Can you work these out from the model? Positions are in its coordinate system, mm. Face numbers are marked on the shaded views. Give positions to 0.01 mm unless a question says otherwise; leave off trailing zeros. Loops run counter-clockwise (first coordinate to the right, second up) from the corner with the lowest first, then second, coordinate; pieces in that order, holes last. Notation, with made-up numbers: M -1,52 L 45,52 A24 cw 45,91 Z; hole C 73,58 d3. An arc over 180 degrees is marked long. One line per item, written item: value. Start each with the question number.
Autodesk Inventor part; units mm, degrees
ref_plane "YZ Plane" through (0, 0, 0) normal (1, 0, 0) x (0, 1, 0)
ref_plane "XZ Plane" through (0, 0, 0) normal (0, 1, 0) x (-1, 0, 0)
ref_plane "XY Plane" through (0, 0, 0) normal (0, 0, 1) x (1, 0, 0)
sketch "Sketch1" plane through (0, 0, 0) normal (0, 1, 0) x (-1, 0, 0)
  circle A0 centre (0, 0) radius 1.05
  line L0 (5, 20) -> (-5, 20)
  line L1 (-5, 20) -> (-5, -5)
  line L2 (-5, -5) -> (5, -5)
  line L3 (5, -5) -> (5, 20)
  circle A1 centre (0, 15) radius 1.05
  dimension "d0" = 2.1
  dimension "d1" = 5
  dimension "d2" = 10
  dimension "d4" = 5
  dimension "d16" = 2.1
  dimension "d17" = 15
  dimension "d18" = 5
extrude "Extrusion1" add sketch "Sketch1" along normal blind 10
sketch "Sketch2" plane through (5, 0, 20) normal (1, 0, 0) x (0, 0, -1)
  line L0 (0, 10) -> (25, 10)
  line L1 (15, 10) -> (17.5478, 3)
  line L2 (17.5478, 3) -> (25, 3)
  line L3 (18.95, 10) -> (18.95, 0)
  line L4 (25, 3) -> (25, 10)
  line L5 (25, 10) -> (15, 10)
  line L6 (25, 0) -> (25, 10)
  line L7 (0, 0) -> (25, 0)
  point P0 (20, 0)
  dimension "d8" = 3
  dimension "d9" = 110
  dimension "d10" = 10
extrude "Extrusion2" cut sketch "Sketch2" against normal blind 10 contours L0 L3 L2 L1 | L0 L4 L2 L3
sketch "Sketch3" plane through (0, 10, 0) normal (0, 1, 0) x (1, 0, 0)
  circle A0 centre (0, 0) radius 2
  dimension "d13" = 4
extrude "Extrusion3" cut sketch "Sketch3" against normal up to surface (7 mm away)
sketch "Sketch4" plane through (0, 10, 0) normal (0, 1, 0) x (1, 0, 0)
  circle A0 centre (0, -15) radius 1.05
  circle A1 centre (0, -15) radius 2.25
  point P0 (0, 0)
  dimension "d19" = 4.5
extrude "Extrusion4" cut sketch "Sketch4" against normal up to surface (7 mm away)
chamfer "Chamfer1" distance 1 angle 45 1 edges at (1.05, 3, 0)
sketch "Sketch5" plane through (5, 0, -5) normal (0, 0, -1) x (-1, 0, 0)
  line L0 (5, 0) -> (5, 5.666) construction
  circle A0 centre (5, 5.666) radius 2.1
  line L1 (10, 3) -> (0, 3)
  dimension "d25" = 4.2
  dimension "d26" = 2.666
extrude "Extrusion5" cut sketch "Sketch5" against normal blind 31.5
sketch "Sketch6" plane through (0, 10, 0) normal (0, 1, 0) x (1, 0, 0)
  line L0 (5, -5) -> (-5, -5)
  line L1 (0, -5) -> (0, -20) construction
  line L2 (-5, -20) -> (5, -20)
  line L3 (3.45, -10.575) -> (-3.45, -10.575)
  line L4 (-3.45, -10.575) -> (-3.45, -7.425)
  line L5 (-3.45, -7.425) -> (3.45, -7.425)
  line L6 (3.45, -7.425) -> (3.45, -10.575)
  line L7 (3.45, -10.575) -> (-3.45, -7.425) construction
  line L8 (-3.45, -10.575) -> (3.45, -7.425) construction
  point P0 (0, 0)
  point P1 (0, -9)
  dimension "d29" = 6.9
  dimension "d30" = 3.15
  dimension "d31" = 4
extrude "Extrusion6" cut sketch "Sketch6" against normal blind 5
sketch "Sketch7" plane through (-3.45, 10, 7.425) normal (0, 0, 1) x (1, 0, 0)
  arc A0 (5.4416, -5) -> (1.4584, -5) centre (3.45, -4.334) ccw
  line L0 (3.45, -8.3177) -> (0, -6.3259)
  line L1 (0, -6.3259) -> (0, -2.3421)
  line L2 (0, -2.3421) -> (3.45, -0.3503)
  line L3 (3.45, -0.3503) -> (6.9, -2.3421)
  line L4 (6.9, -2.3421) -> (6.9, -6.3259)
  line L5 (6.9, -6.3259) -> (3.45, -8.3177)
  point P0 (3.45, -10)
  dimension "d34" = 6.9
extrude "Extrusion7" cut sketch "Sketch7" along normal blind 3.15
sketch "Sketch8" plane through (-5, 0, 20) normal (0, 0, 1) x (1, 0, 0)
  line L0 (0, 10) -> (10, 10)
  line L1 (10, 10) -> (10, 8)
  line L2 (10, 8) -> (0, 8)
  line L3 (0, 8) -> (0, 10)
  line L4 (0, 10) -> (10, 10)
  line L5 (10, 0) -> (10, 10)
  line L6 (0, 0) -> (0, 10)
  point P0 (5, 0)
  dimension "d37" = 2
extrude "Extrusion8" add sketch "Sketch8" along normal blind 28
chamfer "Chamfer2" distance 4 angle 45 1 edges at (0, 8, 20)
sketch "Sketch9" plane through (0, 10, 0) normal (0, 1, 0) x (1, 0, 0)
  circle A0 centre (0, -45) radius 1.05
  line L0 (5, -48) -> (-5, -48)
  point P0 (0, 0)
  dimension "d46" = 2.1
  dimension "d50" = 3
extrude "Extrusion9" cut sketch "Sketch9" against normal blind 15
sketch "Sketch10" plane through (0, 10, 0) normal (0, 1, 0) x (1, 0, 0)
  line L0 (5, -48) -> (-5, -48)
  line L1 (-1.3, -48) -> (-5, -33)
  line L2 (-5, -5) -> (-5, -48)
  line L3 (-5, -33) -> (-5, -48)
  line L4 (-5, -48) -> (-1.3, -48)
  line L5 (0, -35) -> (0, 5) construction
  line L6 (1.3, -48) -> (5, -33)
  line L7 (5, -33) -> (5, -48)
  line L8 (5, -48) -> (1.3, -48)
  point P0 (0, 0)
  dimension "d51" = 1.3
  dimension "d52" = 15
extrude "Extrusion10" cut sketch "Sketch10" against normal blind 15
sketch "Sketch11" plane through (0, 10, 0) normal (0, 1, 0) x (1, 0, 0)
  line L0 (-5, 5) -> (-5, -20)
  line L1 (-5, 5) -> (5, 5)
  line L2 (5, 5) -> (5, -38)
  line L3 (5, -38) -> (-5, -38)
  line L4 (-5, -38) -> (-5, 5)
  line L5 (1.3, -48) -> (-1.3, -48)
  line L6 (5, -5) -> (5, -33)
  point P0 (0, 0)
  dimension "d55" = 10
extrude "Extrusion11" cut sketch "Sketch11" against normal blind 10
properties part number "Clamp"
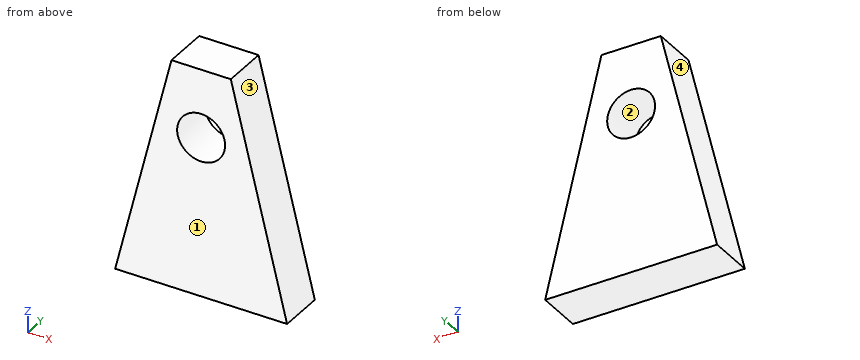
Q1. If we mould it in two halves opening along X, with no side actions, what happens to the marked faces 1, 2, 3 and 4? For each: released by +X, released by -X, zero draft, split by the parting line, or undercut.
Q2. I need wall thicknesses on line 1 along Z through (x, y) = (0, 9.15); line 2 along X through (y, z) = (9.35, 45); line 3 along X through (y, z) = (9.45, 41). Which ranges of each line are inside material? Lowest first, please.
Q3. If we section it at D-D, the plane z = 42: Write out the boundary of the cut face in (x, y).
Q4. If we section it at B-B, the plane x = 0: Write out the boundary of the cut face in (y, z), plus the area to 3 significant figures.
Q5. If we section it at C-C, the plane y = 9.4: Write out the boundary of the cut face in (x, z), plus the area to 3 significant figures.
Q6. If we section it at A-A, the plane z = 45: Write out the boundary of the cut face in (x, y), plus the area to 3 significant figures.
Response:
1. face 1: zero draft
1. face 2: undercut
1. face 3: released by +X
1. face 4: released by -X
2. line 1: 38 to 43.95, 46.05 to 48
2. line 2: -2.04 to -1.05, 1.05 to 2.04
2. line 3: -3.03 to 3.03
3. outline: M -2.78,8 L 2.78,8 L 2.78,10 L -2.78,10 Z
4. outline: M 8,38 L 10,38 L 10,43.95 L 8,43.95 Z; M 8,46.05 L 10,46.05 L 10,48 L 8,48 Z
4. area: 15.8 mm^2
5. outline: M -3.77,38 L 3.77,38 L 1.3,48 L -1.3,48 Z; hole C 0,45 d2.1
5. area: 47.2 mm^2
6. outline: M -2.04,8 L -1.05,8 L -1.05,10 L -2.04,10 Z; M 1.05,8 L 2.04,8 L 2.04,10 L 1.05,10 Z
6. area: 3.96 mm^2
